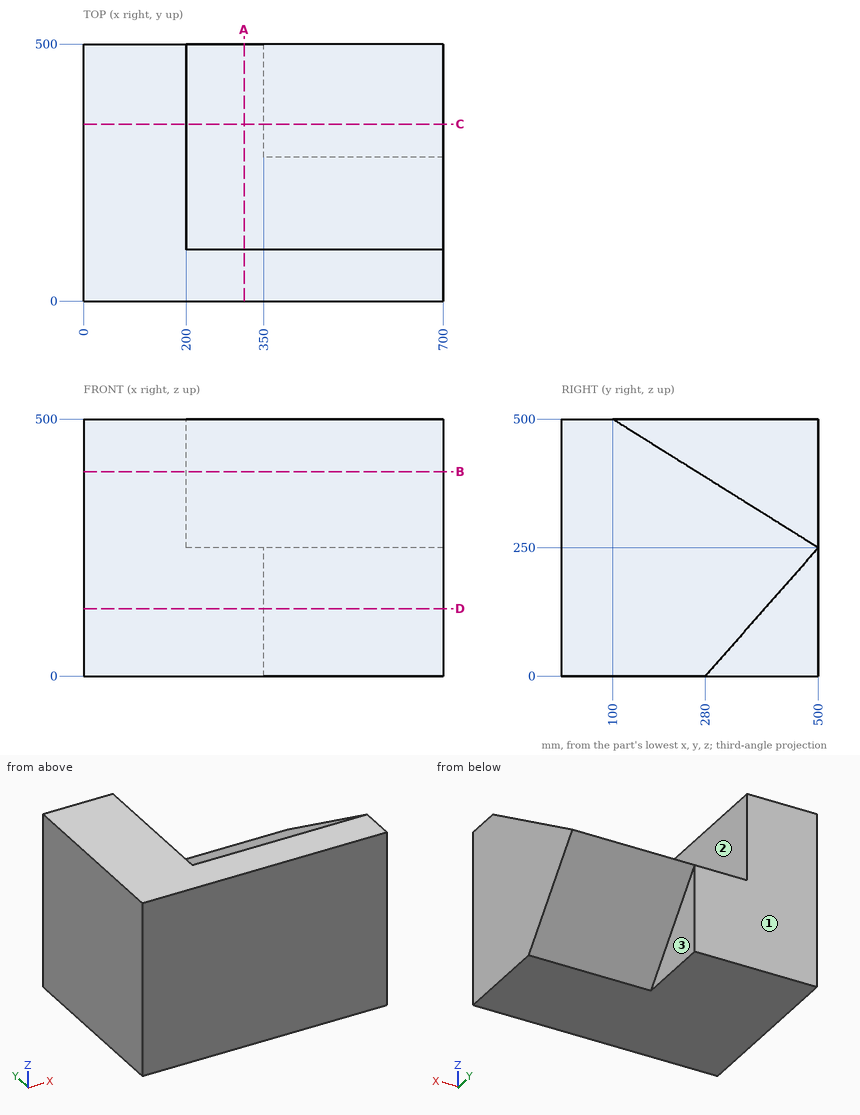
Geometry: see drawing. Coordinates: mm, zero at the bounding-box minimum. A direction names the side the tool comes from. Give positions to 0.01 mm unless a question says otherwise; leave off trailing zeros. Write each loop counter-clockwise with the first axis right and the second up, starting at its lowest first coordinate (ties: lowest second). Pieces come first, ordered by that corner, then holes. Notation, with made-up numbers: M -23,64 L 3,64 A32 cw 3,101 Z; hole C 46,-5.5 d11. An arc over 180 degrees is marked long. Answer in a Markdown table with one row per item. Add a question column.
(1) Section D-D on z = 131. Return loops of the section in (x, y), and give its area (3 significant figures).
(2) First-contact query: pin 1 (8 mm diameter, centred on x = 608.5, z = 440, fed in from -Y); pin 2 (5 mm diameter, centred on x = 527.5, y = 252, fed in from +Z); pin 3 (6 mm diameter, centred on x = 627.5, y = 413.5, fed in from -Z). Flat tips, straight axial feed; report the tip coordinate or a pass-through.
(3) Section B-B on z = 397.5. Return loops of the section in (x, y), and give its area (3 significant figures).
(4) Reachability of the marked faces 1, 2 and 3 from +Z, -Z, +X, -X, +Y, -Y: full face, straight path, thin tool, end or side. Return the list, or none.
(5) Ray query, line 1 (X direction, y = 471.5, z = 444); line 2 (X direction, y = 435.5, z = 146.5); line 3 (Y direction, x = 352.5, z = 233). Return the intervals inside material, ascending.
(6) Section C-C on y = 344. Return loops of the section in (x, z), and give its area (3 significant figures).
(7) Section A-A on x = 312.5. Return loops of the section in (y, z).
Result set:
| question | item | result |
|---|---|---|
| 1 | outline | M 0,0 L 700,0 L 700,395.28 L 350,395.28 L 350,500 L 0,500 Z |
| 1 | area | 313,000 mm^2 |
| 2 | pin 1 | stops at y = 0 |
| 2 | pin 2 | stops at z = 406.56 |
| 2 | pin 3 | stops at z = 148.3 |
| 3 | outline | M 0,0 L 700,0 L 700,264 L 200,264 L 200,500 L 0,500 Z |
| 3 | area | 232,000 mm^2 |
| 4 | face 1 | +Z, -Z, +X, -X, +Y |
| 4 | face 2 | +Z, +X, +Y |
| 4 | face 3 | -Z, +X, +Y |
| 5 | line 1 | x = 0 to 200 |
| 5 | line 2 | x = 0 to 350 |
| 5 | line 3 | y = 0 to 485.04 |
| 6 | outline | M 0,0 L 350,0 L 350,72.73 L 700,72.73 L 700,347.5 L 200,347.5 L 200,500 L 0,500 Z |
| 6 | area | 248,000 mm^2 |
| 7 | outline | M 0,0 L 500,0 L 500,250 L 100,500 L 0,500 Z |
